```python
from build123d import *

# Parameters (mm, degrees)
SKETCH_2_OUTSIDE_W  = 16.94
SKETCH_2_OUTSIDE_H  = 16.94
CUT_EXTRUDE_1_DEPTH = 2.8
CHAMFER_1_SIZE      = 0.4
FILLET_1_R          = 0.4


with BuildPart() as part:
    # Эскиз1 → Повернуть1 (revolve)
    with BuildSketch(Plane(origin=(0, 0, 0), x_dir=(1, 0, 0), z_dir=(0, 1, 0))):
        Polygon((0, 0), (-4, 0), (-4, 2.8), (-2, 2.8), (-2, 32.8), (0, 32.8), align=None)
    revolve(axis=Axis((0, 0, -32.8), (0, 0, 1)))

    # Эскиз2 outside → Вырез-Вытянуть1 (cut)
    with BuildSketch(Plane.XY):
        Rectangle(SKETCH_2_OUTSIDE_W, SKETCH_2_OUTSIDE_H)
        Polygon((0, 3.83), (-3.316877296, 1.915), (-3.316877296, -1.915), (0, -3.83), (3.316877296, -1.915), (3.316877296, 1.915), align=None, mode=Mode.SUBTRACT)
    extrude(amount=-CUT_EXTRUDE_1_DEPTH, mode=Mode.SUBTRACT)

    # Эскиз3 → Вырез-Повернуть1 (revolve, cut)
    with BuildSketch(Plane(origin=(0, 0, 0), x_dir=(0, 0, -1), z_dir=(1, 0, 0))):
        Polygon((0, 3.83), (0.291561886, 3.83), (0, 3.325), align=None)
    revolve(axis=Axis((0, 0, 0), (0, 0, 1)), mode=Mode.SUBTRACT)

    # Фаска1
    chamfer_1_edges = [part.edges().sort_by_distance(p)[0] for p in [
        (2, 0, -32.8),
    ]]
    chamfer(chamfer_1_edges, length=CHAMFER_1_SIZE)

    # Скругление1
    fillet_1_edges = [part.edges().sort_by_distance(p)[0] for p in [
        (2, 0, -2.8),
    ]]
    fillet(fillet_1_edges, radius=FILLET_1_R)


solid = part.part
```
CAD build for the part. Positions are in the model's coordinates, mm. A direction names the side the tool comes from. Round coordinates to 2 decimals unless told otherwise and drop trailing zeros. Order: outer loops, then holes, each group sorted by start corner. A loop starts at its lowest first (then second) coordinate and runs counter-clockwise, first axis right, second up. Notation, with made-up numbers: (36.25, 8.5) -> (62.25, 8.5) arc R33 cw to (62.25, 46.5) -> close; hole circle Ø11 at (86.25, 7). An arc over 180 degrees is marked (long way). One line per question, with ' | ' between items.
Q1. Drop flat-ended pins along their axis: pin 1 (3 mm diameter, centred on x = -1.5, z = -23.5, fed in from -Y); pin 2 (4 mm diameter, centred on y = -3, z = -25, fed in from -X). Give the stop position or say it passes through.
Completed:
pin 1: stops at y = -2 | pin 2: stops at x = -1.73
Q2. Slice it at A-A (z = -15). Write the cut outline in (x, y).
Completed:
outline: circle Ø4 at (0, 0)
Q3. Which spindle directions (+Z, -Z, +X, -X, +Y, -Y) get a long thin tool onto all of the face, cutting with end or side? Do faces 1 (the flat face through (0.8, 2.5, -2.8)), 2 (the flat face through (-1.635, 2.886, -1.38)). Say none if no direction does.
Completed:
face 1: -Z | face 2: +Z, -Z, -X, +Y
Q4. Probe probe 1 along Z at (x, y) = (-1.5, -2.5); probe 2 along X at (y, z) = (-0.75, -6.5). List the from-to ranges inside material, lowest first.
Completed:
probe 1: z = -2.8 to 0 | probe 2: x = -1.85 to 1.85
